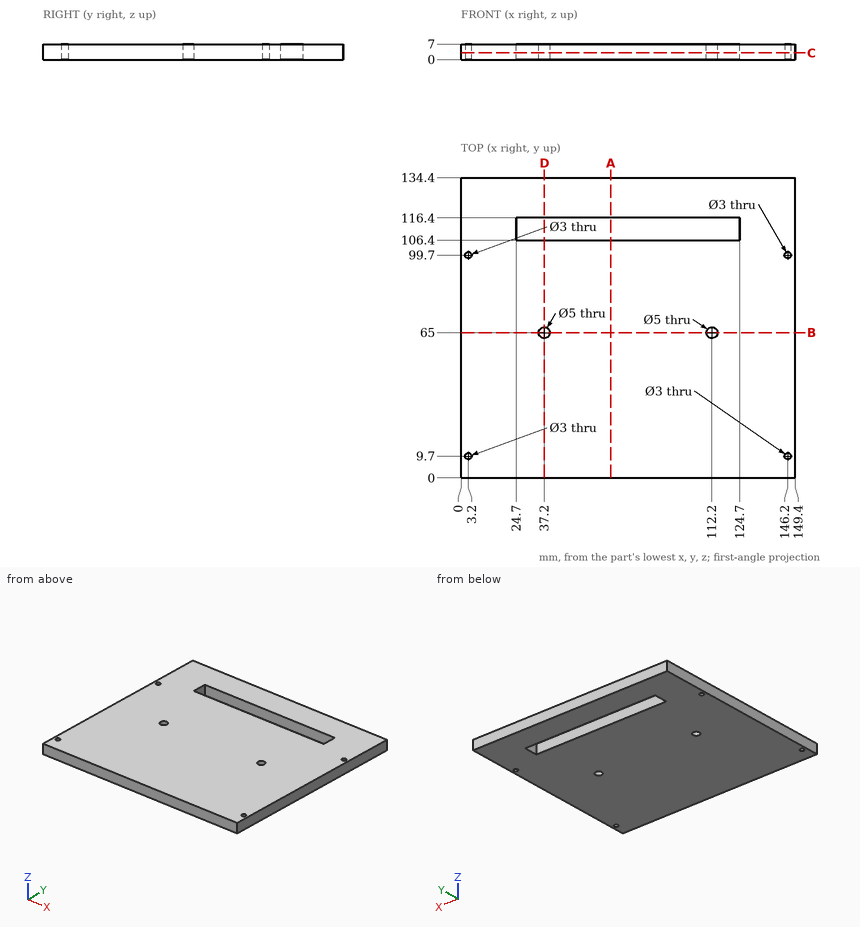
Check sheet for the drawn part. Datum: minimum x, y, z corner. Units: mm. Round coordinates to 2 decimals unless told otherwise and drop trailing zeros. Write each loop counter-clockwise with the first axis right and the second up, starting at its lowest first coordinate (ties: lowest second). Pieces come first, ordered by that corner, then holes. Notation, with made-up numbers: (33, 28.5) -> (51, 28.5) arc R20 cw to (51, 38.5) -> close; hole circle Ø6 at (-16, 24.25). An arc over 180 degrees is marked (long way). Write each question's results on one line, items separated by ' | '. Start each with the question number.
1. Cross-section at D-D (x = 37.2). Enter the section's corners in (y, z), then the cut area to 3 significant figures.
2. Cross-section at B-B (y = 65). Enter the section's corners in (x, z).
3. Cross-section at C-C (z = 3). Enter the section's corners in (x, y).
4. Cross-section at A-A (x = 67). Enter the section's corners in (y, z).
5. Material ranges on probe 1 along Y at (x, z) = (3.2, 1.5); probe 2 along Y at (x, z) = (112.2, 3.75); probe 3 along X at (y, z) = (9.7, 4.5), recorded low to high. Write a range as from..to.
6. Depth check by flat-ended pin: P1, Ø1.8, axis at x = 3.2, y = 99.7, coming from the -Z side. Enter the tip coordinate at first touch or a pass-through.
Solutions:
1) outline: (0, 0) -> (62.5, 0) -> (62.5, 7) -> (0, 7) -> close; (67.5, 0) -> (106.4, 0) -> (106.4, 7) -> (67.5, 7) -> close; (116.4, 0) -> (134.4, 0) -> (134.4, 7) -> (116.4, 7) -> close | area: 836 mm2
2) outline: (0, 0) -> (34.7, 0) -> (34.7, 7) -> (0, 7) -> close; (39.7, 0) -> (109.7, 0) -> (109.7, 7) -> (39.7, 7) -> close; (114.7, 0) -> (149.4, 0) -> (149.4, 7) -> (114.7, 7) -> close
3) outline: (0, 0) -> (149.4, 0) -> (149.4, 134.4) -> (0, 134.4) -> close; hole circle Ø3 at (3.2, 9.7); hole circle Ø3 at (3.2, 99.7); hole (24.7, 106.4) -> (124.7, 106.4) -> (124.7, 116.4) -> (24.7, 116.4) -> close; hole circle Ø5 at (37.2, 65); hole circle Ø5 at (112.2, 65); hole circle Ø3 at (146.2, 9.7); hole circle Ø3 at (146.2, 99.7)
4) outline: (0, 0) -> (106.4, 0) -> (106.4, 7) -> (0, 7) -> close; (116.4, 0) -> (134.4, 0) -> (134.4, 7) -> (116.4, 7) -> close
5) probe 1: y = 0..8.2, 11.2..98.2, 101.2..134.4 | probe 2: y = 0..62.5, 67.5..106.4, 116.4..134.4 | probe 3: x = 0..1.7, 4.7..144.7, 147.7..149.4
6) P1: passes through
